Source: CAD feature listing. Evaluate the final solid. Frame: model axes, mm. Coordinates: 2 decimals unless noted, no trailing zeros. Order: outer loops, then holes, each group sorted by start corner. A loop starts at its lowest first (then second) coordinate and runs counter-clockwise, first axis right, second up. Notation, with made-up numbers: (8, 80.25) - (39, 80.25) arc R18 ccw to (39, 91.25) - close; hole circle Ø9 at (-30, 62.25). An arc over 180 degrees is marked (long way). One line per question, with ' | ' between items. Start each with the question number.
(1) Contact query for flat-ended pins moving along their axis: P1, Ø1.2, axis at x = 4, z = 1.5, coming from the -Y side; P2, Ø1.5, axis at y = 48.5, z = 2.5, coming from the +X side; P3, Ø2, axis at y = -2, z = 2.5, coming from the +X side. Output: stop coordinate, or through.
(2) Section A-A (x = 48.5). Return the cut outline in (y, z).
(3) Line query: line 1 along Y through (x, z) = (40, 0.3); line 2 along X through (y, z) = (49, 3.15); line 3 along Y through (x, z) = (59.5, 1.1). Output: solid intervals per line, ascending.
(4) Section B-B (y = 38). Return the cut outline in (x, z).
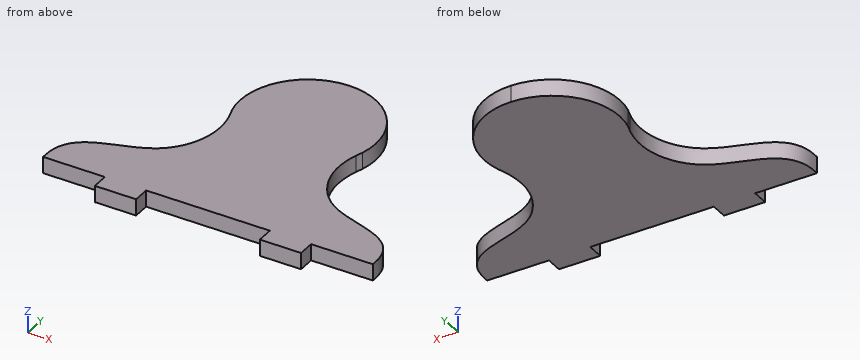
from build123d import *

# Parameters (mm, degrees)
BOSS_EXTRUDE1_DEPTH = 4


with BuildPart() as part:
    # Sketch1 → Boss-Extrude1 (new body)
    with BuildSketch(Plane.XY):
        with BuildLine():
            ThreePointArc((55.819281992, 35.66920927), (53.03910268, 49.949232755), (40, 56.401385036))
            Line((40, 56.401385036), (40, 0))
            Line((40, 0), (55, 0))
            Line((55, 0), (55, -4))
            Line((55, -4), (65, -4))
            Line((65, -4), (65, 0))
            Line((65, 0), (80, 0))
            add(Edge.make_bspline(
                [(80, 0), (80.558151579, 12.429856436), (63.082498357, 9.400795532), (53.987736886, 23.874928316), (54.293563423, 30.674851608), (55.257577446, 33.982379076)],
                knots=[0, 0, 0, 0, 0.197688336, 0.274980814, 0.348282071, 0.348282071, 0.348282071, 0.348282071], degree=3))
            add(Edge.make_bspline(
                [(55.257577446, 33.982379076), (55.421541003, 34.544937251), (55.609085838, 35.107428191), (55.819281992, 35.66920927)],
                knots=[0.348282071, 0.348282071, 0.348282071, 0.348282071, 0.360749457, 0.360749457, 0.360749457, 0.360749457], degree=3))
        make_face()
        with BuildLine():
            add(Edge.make_bspline(
                [(0, 0), (-0.558151579, 12.429856436), (16.917501643, 9.400795532), (26.012263114, 23.874928316), (25.706436577, 30.674851608), (24.742422554, 33.982379076)],
                knots=[0, 0, 0, 0, 0.197688336, 0.274980814, 0.348282071, 0.348282071, 0.348282071, 0.348282071], degree=3))
            Line((0, 0), (15, 0))
            Line((15, 0), (15, -4))
            Line((15, -4), (25, -4))
            Line((25, -4), (25, 0))
            Line((25, 0), (40, 0))
            Line((40, 0), (40, 56.401385036))
            ThreePointArc((40, 56.401385036), (26.96089732, 49.949232755), (24.180718008, 35.66920927))
            add(Edge.make_bspline(
                [(24.742422554, 33.982379076), (24.578458997, 34.544937251), (24.390914162, 35.107428191), (24.180718008, 35.66920927)],
                knots=[0.348282071, 0.348282071, 0.348282071, 0.348282071, 0.360749457, 0.360749457, 0.360749457, 0.360749457], degree=3))
        make_face()
    extrude(amount=BOSS_EXTRUDE1_DEPTH)


solid = part.part
Response values:
1) P1: stops at y = 0 | P2: stops at x = 54.45 | P3: stops at x = 65
2) outline: (0, 0) - (54.03, 0) - (54.03, 4) - (0, 4) - close
3) line 1: y = 0 to 56.4 | line 2: x = 26.29 to 53.71 | line 3: y = -4 to 16.58
4) outline: (23.72, 0) - (56.28, 0) - (56.28, 4) - (23.72, 4) - close
